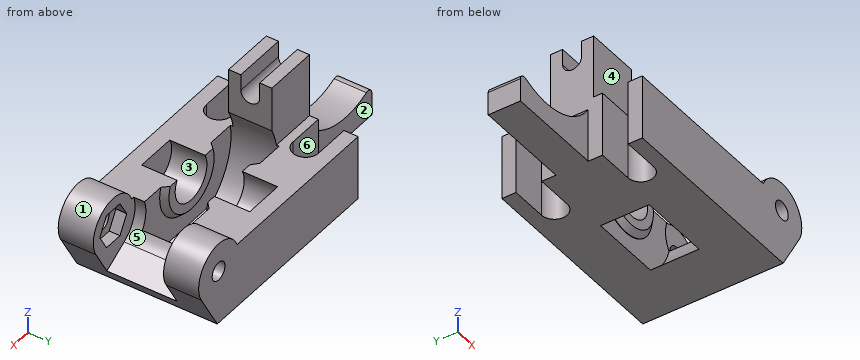
from build123d import *

# Parameters (mm, degrees)
F0_R         = 1.7
F1_DEPTH     = 13
F3_DEPTH     = 12.001
F5_DEPTH     = 6.5
F6_W         = 10
F6_H         = 8
F7_DEPTH     = 11.8
F9_DEPTH     = 42.381
F10_R        = 4.225
F11_DEPTH    = 10
F12_R        = 7.5
F13_DEPTH    = 3.45
F16_R        = 12
F16_R_2      = 6.97
F17_DEPTH    = 4.5
F18_T4_ANGLE = 257.8909092885
F18_T7_ANGLE = 257.8909092885
F20_DEPTH    = 2.9885
F22_DEPTH    = 2


# Not quite as in the source:
# - a fillet or chamfer that OpenCascade refuses, or shapes differently, is made with other operations: its cross-section is extruded or revolved along the edge and cut away or added


with BuildPart() as f1:
    # F0 (on Front) → F1 (new body, symmetric)
    with BuildSketch(Plane.XZ):
        with BuildLine():
            Line((-37.08, 2), (-37.08, -10))
            Line((-37.08, -10), (0.3464101615, -10))
            Line((0.3464101615, -10), (4.5899346401, -2.65))
            ThreePointArc((4.5899346401, -2.65), (2.3304380027, 4.760153224), (-4.9081564767, 2))
            Line((-4.9081564767, 2), (-37.08, 2))
        make_face()
        Circle(F0_R, mode=Mode.SUBTRACT)
    extrude(amount=F1_DEPTH, both=True)

    # F2 (on face) → F3 (cut, through all)
    with BuildSketch(Plane.XY.offset(2)):
        with BuildLine():
            Line((-30.31, 10.385), (-37.08, 10.385))
            Line((-37.08, 10.385), (-37.08, 5.625))
            Line((-37.08, 5.625), (-30.31, 5.625))
            ThreePointArc((-30.31, 5.625), (-27.93, 8.005), (-30.31, 10.385))
        make_face()
        with BuildLine():
            ThreePointArc((-30.31, -10.385), (-27.93, -8.005), (-30.31, -5.625))
            Line((-30.31, -5.625), (-37.08, -5.625))
            Line((-37.08, -5.625), (-37.08, -10.385))
            Line((-37.08, -10.385), (-30.31, -10.385))
        make_face()
    extrude(amount=-F3_DEPTH, mode=Mode.SUBTRACT)

    # F4 (on Front) → F5 (cut, symmetric)
    with BuildSketch(Plane.XZ):
        with BuildLine():
            Line((5.8, -10.0458946839), (5.8, 0))
            ThreePointArc((5.8, 0), (-2.9, 5.0229473419), (-2.9, -5.0229473419))
            Line((-2.9, -5.0229473419), (5.8, -10.0458946839))
        make_face()
    extrude(amount=F5_DEPTH, both=True, mode=Mode.SUBTRACT)

    # F6 (on face) → F7 (join)
    with BuildSketch(Plane.XY.offset(2)):
        with Locations((-32.08, 0)):
            Rectangle(F6_W, F6_H)
    extrude(amount=F7_DEPTH)

    # F8 (on face) → F9 (cut, through all)
    with BuildSketch(Plane(origin=(-37.08, 0, 0), x_dir=(0, -1, 0), z_dir=(-1, 0, 0))):
        with BuildLine():
            Line((1.75, 13.8), (-1.75, 13.8))
            Line((-1.75, 13.8), (-1.75, 10.8))
            ThreePointArc((-1.75, 10.8), (0, 9.05), (1.75, 10.8))
            Line((1.75, 10.8), (1.75, 13.8))
        make_face()
    extrude(amount=-F9_DEPTH, mode=Mode.SUBTRACT)

    # F10 (on Front) → F11 (cut, symmetric)
    with BuildSketch(Plane.XZ):
        with Locations((-16.3, 0)):
            Circle(F10_R)
    extrude(amount=F11_DEPTH, both=True, mode=Mode.SUBTRACT)

    # F12 (on Front) → F13 (cut, symmetric)
    with BuildSketch(Plane.XZ):
        with Locations((-16.3, 0)):
            Circle(F12_R)
    extrude(amount=F13_DEPTH, both=True, mode=Mode.SUBTRACT)

    # F16 (on Front) → F17 (cut, symmetric)
    with BuildSketch(Plane.XZ):
        with Locations((-16.4292231202, 0)):
            Circle(F16_R)
        with Locations((-16.4292231202, 0)):
            Circle(F16_R_2, mode=Mode.SUBTRACT)
    extrude(amount=F17_DEPTH, both=True, mode=Mode.SUBTRACT)

    # F18: chamfer of 1.05 x 0.9699305265 on 2 edges, made by hand


with BuildPart() as f18_tool2:
    # F18_s3 → F18_t4 (revolve)
    with BuildSketch(Plane(origin=(-6.4914021144, 0, -8.0318361717), x_dir=(0, 1, 0), z_dir=(0.6285802661, 0, 0.7777447197))):
        Polygon((-3.45, 18.7778110045), (-4.5, 19.747741531), (-3.45, 19.747741531), align=None)
    revolve(axis=Axis((-16.4292231202, -3.45, 0), (0, -1, 0)), revolution_arc=F18_T4_ANGLE)

    split(bisect_by=Plane.XZ.offset(4.5), keep=Keep.BOTTOM)


with BuildPart() as f1_1:
    add(f1.part)

    # F18_t1: cut F18_tool2
    add(f18_tool2.part, mode=Mode.SUBTRACT)

    # F18_s6 → F18_t7 (revolve, cut)
    with BuildSketch(Plane(origin=(-6.4914021144, 0, 8.0318361717), x_dir=(0, 1, 0), z_dir=(-0.6285802661, 0, 0.7777447197))):
        Polygon((4.4199305265, 5.807741531), (3.45, 6.857741531), (3.45, 5.807741531), align=None)
    revolve(axis=Axis((-16.4292231202, 3.45, 0), (0, 1, 0)), revolution_arc=F18_T7_ANGLE, mode=Mode.SUBTRACT)

    # F19 (on Front) → F20 (join, symmetric)
    with BuildSketch(Plane.XZ):
        with BuildLine():
            Line((-37.08, -10), (-37.08, 0))
            ThreePointArc((-37.08, 0), (-44.4762536163, -5.4872309342), (-53.6579068221, -4.7720279633))
            ThreePointArc((-53.6579068221, -4.7720279633), (-54.617543869, -4.8353446309), (-55.08, -5.6785804158))
            Line((-55.08, -5.6785804158), (-55.08, -10))
            Line((-55.08, -10), (-37.08, -10))
        make_face()
    extrude(amount=F20_DEPTH, both=True)

    # F21 (on face) → F22 (cut)
    with BuildSketch(Plane(origin=(0, -6.5, 0), x_dir=(-1, 0, 0), z_dir=(0, 1, 0))):
        Polygon((-3.579571669, 0), (-1.7897858345, -3.1), (1.7897858345, -3.1), (3.579571669, 0), (1.7897858345, 3.1), (-1.7897858345, 3.1), align=None)
    extrude(amount=-F22_DEPTH, mode=Mode.SUBTRACT)


solid = f1_1.part
The listing builds one solid part. Answer for the finished solid, in the listing's coordinates (mm). Face numbers are marked on the shaded views. A direction names the side the tool comes from. Coordinates: 2 decimals unless noted, no trailing zeros. Write each loop counter-clockwise with the first axis right and the second up, starting at its lowest first coordinate (ties: lowest second). Pieces come first, ordered by that corner, then holes. Notation, with made-up numbers: M -40,66 L -25,66 A19 cw -25,96 Z; hole C 53.5,31.5 d8. An arc over 180 degrees is marked long. Write each question's results on one line, items separated by ' | '.
Item 1: The part is cut by section B-B on x = -0.5. Determine the outline of the cut face in (y, z), and give its area (3 significant figures).
Answer below:
outline: M -13,-10 L 13,-10 L 13,-1.62 L 6.5,-1.62 L 6.5,-6.41 L -6.5,-6.41 L -6.5,-3.1 L -8.5,-3.1 L -8.5,-1.62 L -13,-1.62 Z; M -13,1.62 L -8.5,1.62 L -8.5,3.1 L -6.5,3.1 L -6.5,5.28 L -13,5.28 Z; M 6.5,1.62 L 13,1.62 L 13,5.28 L 6.5,5.28 Z | area: 197 mm2
Item 2: The part is cut by section C-C on y = 0. Determine the outline of the cut face in (x, z).
Answer below:
outline: M -55.08,-10 L -23.06,-10 A12 cw -27.08,5.53 L -27.08,9.05 L -37.08,9.05 L -37.08,0 A13.14 cw -53.66,-4.77 A1 ccw -55.08,-5.68 Z; M -9.8,-10 L 0.35,-10 L 1.69,-7.67 L -2.9,-5.02 A5.8 cw -4.86,-3.17 A12 cw Z
Item 3: Consider probe 1 along Y at (x, z) = (-33, 1.25) (3 decimals); probe 2 along Z at (x, y) = (0, -11.95); probe 3 along Y at (x, z) = (-14.5, 0). Determine where each line is inside the solid, lowest interval first. Write a range as [from, to].
Answer below:
probe 1: [-13, -10.385], [-5.625, 5.625], [10.385, 13] | probe 2: [-10, -1.7], [1.7, 5.3] | probe 3: [-13, -10], [10, 13]
Item 4: Which of the six approach directions +Z, -Z, +X, -X, +Y, -Y give full straight-line access (tool end or side, diameter ignored) to the marked faces 4, 5 and 6?
Answer below:
face 4: +Z, +X, -X, -Y | face 5: +X | face 6: +Z, -Z, -X
Item 5: The part is cut by section A-A on y = 8. Determine the outline of the cut face in (x, z) (3 decimals).
Answer below:
outline: M -27.93,-10 L 0.346,-10 L 4.59,-2.65 A5.3 ccw long -4.908,2 L -12.578,2 A4.225 cw long -20.022,2 L -27.93,2 Z; hole C 0,0 d3.4
Item 6: For a pull along Y with two mould halves and no side action, classify the marked faces 1, 2 and 3 as released by +Y, released by -Y, zero draft, split by the parting line, or undercut.
Answer below:
face 1: zero draft | face 2: released by +Y | face 3: undercut
Item 7: The part is cut by section D-D on z = -8.5. Determine the outline of the cut face in (x, y) (1 decimal), and give its area (3 significant figures).
Answer below:
outline: M -55.1,-3 L -37.1,-3 L -37.1,-5.6 L -30.3,-5.6 A2.4 cw -30.3,-10.4 L -37.1,-10.4 L -37.1,-13 L 1.2,-13 L 1.2,13 L -37.1,13 L -37.1,10.4 L -30.3,10.4 A2.4 cw -30.3,5.6 L -37.1,5.6 L -37.1,3 L -55.1,3 Z; hole M -24.9,-4.5 L -8,-4.5 L -8,4.5 L -24.9,4.5 Z | area: 868 mm2
Item 8: Given P1, Ø0.9, axis at x = -34, z = 13, coming from the -Y side; P2, Ø3, axis at x = -22.5, y = 8.5, coming from the +Z side; P3, Ø2, axis at y = -12, z = -2, coming from the -X side, each flat-ended and moving along its own axis, determine where each tip first touches the part or whether it passes through.
Answer below:
P1: y = -4 | P2: z = 2 | P3: x = -37.08
